Here's the drawing with two shaded views (mm, measured from the low corner). I have some questions. A direction names the side the tool comes from. Give positions to 0.01 mm unless a question says otherwise; leave off trailing zeros. Write each loop counter-clockwise with the first axis right and the second up, starting at its lowest first coordinate (ties: lowest second). Pieces come first, ordered by that corner, then holes. Notation, with made-up numbers: (-26.5, -20.5) -> (-1.5, -20.5) arc R9 ccw to (-1.5, -7.5) -> close; hole circle Ø6 at (12.5, -4.5). An arc over 180 degrees is marked (long way). One line per item, written item: value.
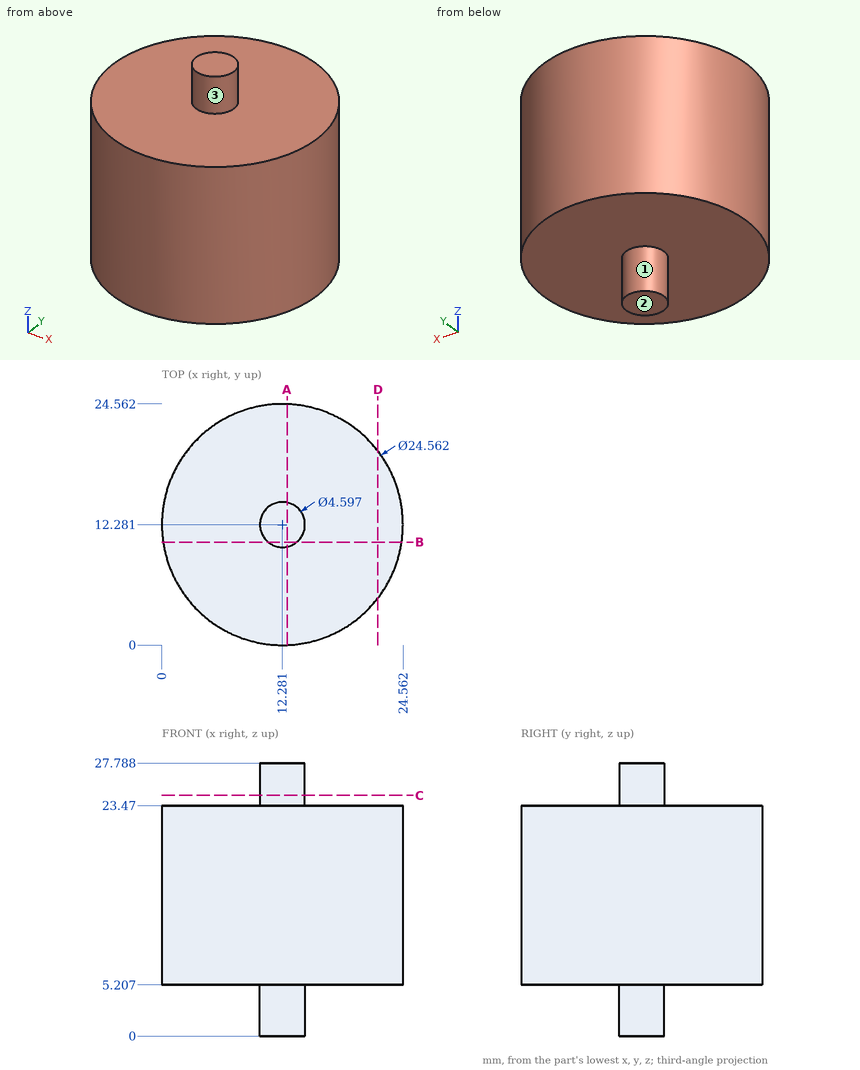
1) Will these pins go through, and if not, where does the flat tip stop? pin 1 (2 mm diameter, centred on x = 9, y = 21.5, fed in from -Z); pin 2 (8 mm diameter, centred on x = 8, z = 18, fed in from +Y); pin 3 (2 mm diameter, centred on x = 17, z = 16.5, fed in from +Y) (1 decimal).
Answer list:
pin 1: stops at z = 5.21
pin 2: stops at y = 24.56
pin 3: stops at y = 24
2) For the marked faces 1, 2 and 3, which set-ups out of +Z, -Z, +X, -X, +Y, -Y let a thin tool reach every point of the face, with its end or its side?
Answer list:
face 1: -Z
face 2: -Z, +X, -X, +Y, -Y
face 3: +Z
3) If we section it at C-C (z = 24.5): Write out the boundary of the cut face in (x, y).
Answer list:
outline: circle Ø4.6 at (12.28, 12.28)
4) I need wall thicknesses on L1, parallel to Z at x = 23, y = 9.5; L2, parallel to Y at x = 2.25, z = 9.25 (1 decimal); L3, parallel to Y at x = 2, z = 8.5 (1 decimal). Which ranges of each line are inside material? Lowest first, please.
Answer list:
L1: z = 5.21 to 23.47
L2: y = 5.2 to 19.4
L3: y = 5.6 to 19
5) If we section it at A-A (x = 12.75): Write out the boundary of the cut face in (y, z), and give its area (3 significant figures).
Answer list:
outline: (0.01, 5.21) -> (10.03, 5.21) -> (10.03, 0) -> (14.53, 0) -> (14.53, 5.21) -> (24.55, 5.21) -> (24.55, 23.47) -> (14.53, 23.47) -> (14.53, 27.79) -> (10.03, 27.79) -> (10.03, 23.47) -> (0.01, 23.47) -> close
area: 491 mm^2
6) If we section it at B-B (y = 10.5): Write out the boundary of the cut face in (x, z) (1 decimal).
Answer list:
outline: (0.1, 5.2) -> (10.8, 5.2) -> (10.8, 0) -> (13.7, 0) -> (13.7, 5.2) -> (24.4, 5.2) -> (24.4, 23.5) -> (13.7, 23.5) -> (13.7, 27.8) -> (10.8, 27.8) -> (10.8, 23.5) -> (0.1, 23.5) -> close
7) If we section it at D-D (x = 22): Write out the boundary of the cut face in (y, z).
Answer list:
outline: (4.77, 5.21) -> (19.79, 5.21) -> (19.79, 23.47) -> (4.77, 23.47) -> close
